from build123d import *

# Parameters (mm, degrees)
F2_SIZE = 0.5


with BuildPart() as f1:
    # F0 (on Front) → F1 (revolve)
    with BuildSketch(Plane.XZ):
        with BuildLine():
            Line((0, 5.365184), (0, 0))
            Line((0, 0), (3.95, 0))
            Line((3.95, 0), (3.95, 3.4))
            Line((3.95, 3.4), (7, 3.4))
            Line((7, 3.4), (7, 3.9))
            ThreePointArc((7, 3.9), (7.292893, 4.607107), (8, 4.9))
            Line((8, 4.9), (10.5, 4.9))
            ThreePointArc((10.5, 4.9), (11.207107, 5.192893), (11.5, 5.9))
            ThreePointArc((11.5, 5.9), (11.207107, 6.607107), (10.5, 6.9))
            Line((10.5, 6.9), (9.817803, 6.9))
            ThreePointArc((9.817803, 6.9), (9.508896, 6.876), (9.207402, 6.804576))
            ThreePointArc((9.207402, 6.804576), (4.659616, 5.727204), (0, 5.365184))
        make_face()
    revolve(axis=Axis((0, 0, 2.682592), (0, 0, -1)))

    # F2
    f2_edges = [f1.edges().sort_by_distance(p)[0] for p in [
        (-3.95, 0, 0),
    ]]
    chamfer(f2_edges, length=F2_SIZE)


solid = f1.part
Read the model definition and answer for the solid it produces. Units are mm, in the model's axes. A direction names the side the tool comes from. Coordinates: 2 decimals unless noted, no trailing zeros. Put each result on its own line as item: value. Start each with the question number.
Item 1: For faces 1 (the face through (6, 8, 6.9)), 2 (the face through (2, 8, 4.9)), determine the directions among +Z, -Z, +X, -X, +Y, -Y from which every point of the face is accessible in a straight line to the end or side of a thin tool.
Item 2: Given pin 1 Ø4 at (y, z) = (-9, 1.5) entering from +X; pin 2 Ø1.5 at (y, z) = (-6, 3) entering from +X; pin 3 Ø8 at (x, y) = (-8, -8.5) entering from -Z; pin 4 Ø4 at (x, y) = (-1, 6) entering from -Z, each flat-ended and moving along its own axis, determine where each tip first touches the part or whether it passes through.
Item 3: Consider probe 1 along Z at (x, y) = (5, -9); probe 2 along Y at (x, z) = (-2.25, 4.5); probe 3 along Z at (x, y) = (6.25, 2.5). Determine where each line is inside the solid, lowest interval first. Write a range as [from, to].
Computed:
1. face 1: +Z, +X, -X, +Y, -Y
1. face 2: -Z
2. pin 1: passes through
2. pin 2: stops at x = 4.5
2. pin 3: stops at z = 4.84
2. pin 4: stops at z = 3.4
3. probe 1: z = [4.9, 6.9]
3. probe 2: y = [-6.84, 6.84]
3. probe 3: z = [3.4, 6.13]
